Geometry: final body of the model. Coordinates: model frame, mm. Coordinates: 2 decimals unless noted, no trailing zeros. Order: outer loops, then holes, each group sorted by start corner. A loop starts at its lowest first (then second) coordinate and runs counter-clockwise, first axis right, second up. Notation, with made-up numbers: M 12.5,89 L 63.5,89 A7 cw 63.5,100 Z; hole C -0.5,37.25 d8. An arc over 180 degrees is marked long. One line per question, with ' | ' between items.
from build123d import *

# Parameters (mm, degrees)
SKETCH1_W           = 120
SKETCH1_H           = 170
SKETCH1_R           = 2.65
SKETCH1_R_2         = 2.5
SKETCH1_R_3         = 3
BOSS_EXTRUDE1_DEPTH = 5
FILLET1_R           = 0.5


with BuildPart() as part:
    # Sketch1 → Boss-Extrude1 (new body)
    with BuildSketch(Plane.XY):
        with Locations((60, 85)):
            Rectangle(SKETCH1_W, SKETCH1_H)
        with Locations((28, 22)):
            Circle(SKETCH1_R, mode=Mode.SUBTRACT)
        with Locations((7, 22)):
            Circle(SKETCH1_R, mode=Mode.SUBTRACT)
        with Locations((7, 50)):
            Circle(SKETCH1_R, mode=Mode.SUBTRACT)
        with Locations((28, 50)):
            Circle(SKETCH1_R, mode=Mode.SUBTRACT)
        with Locations((28, 121)):
            Circle(SKETCH1_R, mode=Mode.SUBTRACT)
        with Locations((7, 121)):
            Circle(SKETCH1_R, mode=Mode.SUBTRACT)
        with Locations((28, 149)):
            Circle(SKETCH1_R, mode=Mode.SUBTRACT)
        with Locations((7, 149)):
            Circle(SKETCH1_R, mode=Mode.SUBTRACT)
        with Locations((39, 22.5)):
            Circle(SKETCH1_R_2, mode=Mode.SUBTRACT)
        with Locations((81, 22.5)):
            Circle(SKETCH1_R_2, mode=Mode.SUBTRACT)
        with Locations((5, 163)):
            Circle(SKETCH1_R_3, mode=Mode.SUBTRACT)
        with Locations((115, 163)):
            Circle(SKETCH1_R_3, mode=Mode.SUBTRACT)
        with Locations((37, 163)):
            Circle(SKETCH1_R_3, mode=Mode.SUBTRACT)
        with Locations((83, 163)):
            Circle(SKETCH1_R_3, mode=Mode.SUBTRACT)
        with Locations((115, 7)):
            Circle(SKETCH1_R_3, mode=Mode.SUBTRACT)
        with Locations((83, 7)):
            Circle(SKETCH1_R_3, mode=Mode.SUBTRACT)
        with Locations((37, 7)):
            Circle(SKETCH1_R_3, mode=Mode.SUBTRACT)
        with Locations((5, 7)):
            Circle(SKETCH1_R_3, mode=Mode.SUBTRACT)
        with Locations((39, 145.5)):
            Circle(SKETCH1_R_2, mode=Mode.SUBTRACT)
        with Locations((81, 145.5)):
            Circle(SKETCH1_R_2, mode=Mode.SUBTRACT)
        with Locations((113, 149)):
            Circle(SKETCH1_R, mode=Mode.SUBTRACT)
        with Locations((92, 149)):
            Circle(SKETCH1_R, mode=Mode.SUBTRACT)
        with Locations((92, 121)):
            Circle(SKETCH1_R, mode=Mode.SUBTRACT)
        with Locations((113, 121)):
            Circle(SKETCH1_R, mode=Mode.SUBTRACT)
        with Locations((92, 50)):
            Circle(SKETCH1_R, mode=Mode.SUBTRACT)
        with Locations((113, 50)):
            Circle(SKETCH1_R, mode=Mode.SUBTRACT)
        with Locations((113, 22)):
            Circle(SKETCH1_R, mode=Mode.SUBTRACT)
        with Locations((92, 22)):
            Circle(SKETCH1_R, mode=Mode.SUBTRACT)
        with Locations((109, 97.5)):
            Circle(SKETCH1_R_2, mode=Mode.SUBTRACT)
        with Locations((109, 73.5)):
            Circle(SKETCH1_R_2, mode=Mode.SUBTRACT)
        with Locations((91, 73.5)):
            Circle(SKETCH1_R_2, mode=Mode.SUBTRACT)
        with Locations((91, 97.5)):
            Circle(SKETCH1_R_2, mode=Mode.SUBTRACT)
    extrude(amount=BOSS_EXTRUDE1_DEPTH)

    # Fillet1
    fillet1_edges = [part.edges().sort_by_distance(p)[0] for p in [
        (120, 0, 2.5),
        (0, 0, 2.5),
    ]]
    fillet(fillet1_edges, radius=FILLET1_R)


solid = part.part
1. Draft query along Y for faces 1 (the face through (120, 84, 2)), 2 (the face through (59, 170, 2)), 3 (the face through (80, 7, 2)). Return one class per face: pulls with the +Y half, pulls with the -Y half, needs draft (parallel to the pull), parting line crosses it, or undercut.
Response values:
face 1: needs draft | face 2: pulls with the +Y half | face 3: undercut
2. Pin query (flat end, axial travel): P1, Ø1, axis at x = 33.5, y = 148.5, coming from the -Z side. Return the tip coordinate at first contact, or that it passes through.
Response values:
P1: stops at z = 0
3. Section A-A, the plane y = 73.5. Output: boundary loops of the cut face in (x, z).
Response values:
outline: M 0,0 L 88.5,0 L 88.5,5 L 0,5 Z; M 93.5,0 L 106.5,0 L 106.5,5 L 93.5,5 Z; M 111.5,0 L 120,0 L 120,5 L 111.5,5 Z
4. Section D-D, the plane y = 7. Output: boundary loops of the cut face in (x, z).
Response values:
outline: M 0,0 L 2,0 L 2,5 L 0,5 Z; M 8,0 L 34,0 L 34,5 L 8,5 Z; M 40,0 L 80,0 L 80,5 L 40,5 Z; M 86,0 L 112,0 L 112,5 L 86,5 Z; M 118,0 L 120,0 L 120,5 L 118,5 Z
5. Section C-C, the plane z = 3.75. Give the number of separate pieces and of enclosed holes in the cut face, and give its area (3 significant figures).
Response values:
separate pieces: 1 | enclosed holes: 32 | area: 19,700 mm^2
6. Section B-B, the plane y = 50. Output: boundary loops of the cut face in (x, z).
Response values:
outline: M 0,0 L 4.35,0 L 4.35,5 L 0,5 Z; M 9.65,0 L 25.35,0 L 25.35,5 L 9.65,5 Z; M 30.65,0 L 89.35,0 L 89.35,5 L 30.65,5 Z; M 94.65,0 L 110.35,0 L 110.35,5 L 94.65,5 Z; M 115.65,0 L 120,0 L 120,5 L 115.65,5 Z
7. Material intervals for line 1 (X direction, y = 149, z = 1.7); line 2 (Y direction, x = 107, z = 4.45), sorted ascending. Write a range as [from, to].
Response values:
line 1: x = [0, 4.35], [9.65, 25.35], [30.65, 89.35], [94.65, 110.35], [115.65, 120] | line 2: y = [0, 72], [75, 96], [99, 170]
